For this review, take the finished solid that the model builds, in its own axes (mm). A direction names the side the tool comes from. Coordinates: 2 decimals unless noted, no trailing zeros. Write each loop counter-clockwise with the first axis right and the second up, starting at its lowest first coordinate (ties: lowest second). Pieces come first, ordered by that corner, then holes.
```python
from build123d import *

# Parameters (mm, degrees)
F1_DEPTH = 25
F2_W     = 21
F2_H     = 24
F2_R     = 5.1
F3_DEPTH = 3
F6_DEPTH = 2.95
F8_R     = 1


with BuildPart() as f1:
    # F0 (on Top) → F1 (new body)
    with BuildSketch(Plane.XY):
        with BuildLine():
            ThreePointArc((7.5943561158, -9.0506011845), (7.5880140669, -10.4148995325), (8.8942921325, -10.8085844568))
            ThreePointArc((8.8942921325, -10.8085844568), (14.7842599605, 2.839809495), (6.2367777531, 15.0016731019))
            ThreePointArc((6.2367777531, 15.0016731019), (5.8102691618, 15.8862752393), (6.5779752006, 16.4986949957))
            Line((6.5779752006, 16.4986949957), (10.5, 16.4986949957))
            Line((10.5, 16.4986949957), (10.5, 19.4986949957))
            Line((10.5, 19.4986949957), (-10.5, 19.4986949957))
            Line((-10.5, 19.4986949957), (-10.5, 16.4986949957))
            Line((-10.5, 16.4986949957), (-6.5779752006, 16.4986949957))
            ThreePointArc((-6.5779752006, 16.4986949957), (-5.8102691618, 15.8862752393), (-6.2367777531, 15.0016731019))
            ThreePointArc((-6.2367777531, 15.0016731019), (-14.7842599605, 2.839809495), (-8.8942921325, -10.8085844568))
            ThreePointArc((-8.8942921325, -10.8085844568), (-7.5880140669, -10.4148995325), (-7.5943561158, -9.0506011845))
            ThreePointArc((-7.5943561158, -9.0506011845), (-11.760600173, 4.9065375968), (0, 13.5))
            ThreePointArc((0, 13.5), (11.760600173, 4.9065375968), (7.5943561158, -9.0506011845))
        make_face()
    extrude(amount=F1_DEPTH)

    # F2 (on face) → F3 (join)
    with BuildSketch(Plane.XY.offset(25)):
        with Locations((0, 31.4986949957)):
            Rectangle(F2_W, F2_H)
        with Locations((0, 34.4986949957)):
            Circle(F2_R, mode=Mode.SUBTRACT)
    extrude(amount=-F3_DEPTH)

    # F4: union 

    # F5 (on face) → F6 (join)
    with BuildSketch(Plane.YZ.offset(10.5)):
        Polygon((19.4986949957, 22), (19.4986949957, 0), (43.4986949957, 22), align=None)
    extrude(amount=-F6_DEPTH)

    # F7: F1 across plane


with BuildPart() as f1_1:
    add(f1.part)
    add(f1.part.mirror(Plane.YZ))

    # F8
    f8_edges = [f1_1.edges().sort_by_distance(p)[0] for p in [
        (10.5, 17.998695, 0),
        (10.5, 16.498695, 12.5),
        (10.5, 29.998695, 25),
        (10.5, 43.498695, 23.5),
        (10.5, 31.498695, 11),
        (-10.5, 43.498695, 23.5),
        (-10.5, 29.998695, 25),
        (-10.5, 16.498695, 12.5),
        (-10.5, 17.998695, 0),
        (-10.5, 31.498695, 11),
    ]]
    fillet(f8_edges, radius=F8_R)


solid = f1_1.part
```
Q1. Clearance check with flat-ended pins moving along their axes: pin 1 Ø4 at (y, z) = (33.5, 15) entering from +X; pin 2 Ø10 at (y, z) = (7, 18) entering from +X; pin 3 Ø12 at (x, y) = (-3, 31) entering from -Z. State where each tip first meets the part, or that it passes through.
Ans:
pin 1: stops at x = 10.5
pin 2: stops at x = 14.85
pin 3: stops at z = 6.96
Q2. Tool access review of faces 1 (the flat face through (-10.5, 27, 15)), 2 (the cylindrical face through (-11.83, 4.7, 12.32)), 3 (the flat face through (-8, 16.499, 12)), 4 (the flat face through (8, 16.499, 12)): name each direction out of +Z, -Z, +X, -X, +Y, -Y from which nothing blocks a thin tool from reaching the whole face with its end or side.
Ans:
face 1: +Z, -Z, -X, +Y
face 2: +Z, -Z
face 3: +Z, -Z, -X
face 4: +Z, -Z, +X
Q3. Add section B-B (x = -1.5). State the section outline as (y, z) points.
Ans:
outline: (13.39, 0) - (19.5, 0) - (19.5, 22) - (29.62, 22) - (29.62, 25) - (13.39, 25) - close; (39.37, 22) - (43.5, 22) - (43.5, 25) - (39.37, 25) - close
Q4. Draft analysis for pull direction Y (two halves, no side actions). For faces 5 (the flat face through (-7.55, 29, 14)), 6 (the cylindrical face through (7.576, -10.398, 12.325)), 7 (the cylindrical face through (-10.2, 31.47, 11.36)), 8 (the cylindrical face through (-0.664, 39.555, 23.521)), state which applies: +Y half, -Y half, draft (parallel to the pull), parting line (faces both ways), or undercut.
Ans:
face 5: draft
face 6: undercut
face 7: +Y half
face 8: undercut
Q5. For probe 1 along Y at (x, z) = (0, 24.2); probe 2 along X at (y, z) = (25.5, 12.5); probe 3 along X at (y, z) = (-6.5, 3), list the stretches that pass through material, from the lowest coordinate up.
Ans:
probe 1: y = 13.5 to 29.4, 39.6 to 43.5
probe 2: x = -10.5 to -7.55, 7.55 to 10.5
probe 3: x = -12.73 to -10.04, 10.04 to 12.73
Q6. Add section A-A (y = 10). State the section outline as (x, z) points, then the cut area to 3 significant figures.
Ans:
outline: (-12.12, 0) - (-8.52, 0) - (-8.52, 25) - (-12.12, 25) - close; (8.52, 0) - (12.12, 0) - (12.12, 25) - (8.52, 25) - close
area: 180 mm2
